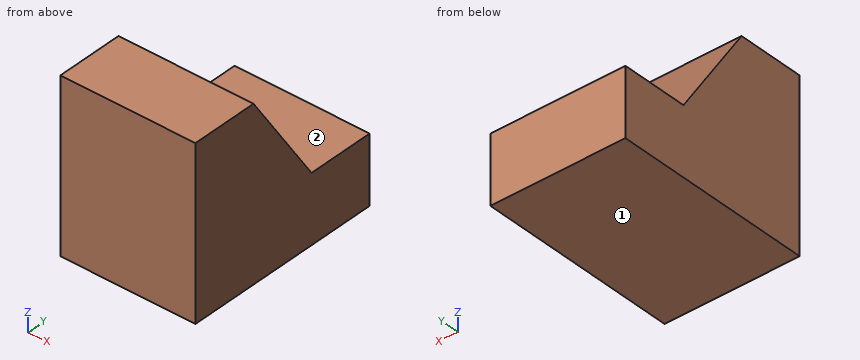
```python
from build123d import *

# Parameters (mm, degrees)
F0_W     = 38.1
F0_H     = 31.75
F1_DEPTH = 25.4
F3_DEPTH = 25.401


with BuildPart() as f1:
    # F0 (on Right) → F1 (new body)
    with BuildSketch(Plane.YZ):
        with Locations((19.05, 15.875)):
            Rectangle(F0_W, F0_H)
    extrude(amount=F1_DEPTH)

    # F2 (on face) → F3 (cut, through all)
    with BuildSketch(Plane.YZ.offset(25.4)):
        Polygon((25.4, 12.7), (38.1, 12.7), (38.1, 31.75), (12.7, 31.75), align=None)
    extrude(amount=-F3_DEPTH, mode=Mode.SUBTRACT)


solid = f1.part
```
Could you check a few things on this model? Use its own coordinates, in mm. Face numbers are marked on the shaded views. A direction names the side the tool comes from. Round coordinates to 2 decimals unless told otherwise and drop trailing zeros. Write each loop counter-clockwise with the first axis right and the second up, starting at its lowest first coordinate (ties: lowest second). Pieces come first, ordered by that corner, then holes.
(1) Suppose I cut it at B-B on y = 15.5. Write out the boundary of the cut face in (x, z).
Findings below:
outline: (0, 0) - (25.4, 0) - (25.4, 27.55) - (0, 27.55) - close
(2) Which directions (+Z, -Z, +X, -X, +Y, -Y) give clear straight access to the entire face, cutting with the end or side of a thin tool? Please do the marked faces 1 and 2.
Findings below:
face 1: -Z, +X, -X, +Y, -Y
face 2: +Z, +X, -X, +Y
(3) Suppose I cut it at A-A on z = 25. Write out the boundary of the cut face in (x, y).
Findings below:
outline: (0, 0) - (25.4, 0) - (25.4, 17.2) - (0, 17.2) - close
(4) Suppose I cut it at C-C on x = 17.25. Write out the boundary of the cut face in (y, z), and give its area (3 significant figures).
Findings below:
outline: (0, 0) - (38.1, 0) - (38.1, 12.7) - (25.4, 12.7) - (12.7, 31.75) - (0, 31.75) - close
area: 847 mm2
(5) For pin 1 (6.5 mm diameter, centred on x = 15, y = 35, fed in from +Z), with a flat end and sliding along its axis, tell me the tip position at first contact or that it passes through.
Findings below:
pin 1: stops at z = 12.7
(6) If I drill on probe 1 along Z at (x, y) = (14.25, 32); probe 2 along Y at (x, z) = (19.5, 26.5); probe 3 along Y at (x, z) = (15.5, 16.5), over which ranges is the centre line in solid material (lowest first)?
Findings below:
probe 1: z = 0 to 12.7
probe 2: y = 0 to 16.2
probe 3: y = 0 to 22.87
